from build123d import *

# Parameters (mm, degrees)
SKETCH1_R               = 5
BOSS_EXTRUDE1_DEPTH     = 5
SKETCH2_R               = 5.5
BOSS_EXTRUDE2_DEPTH     = 0.4
CUT_EXTRUDE1_DEPTH      = 6.4
SKETCH5_R               = 8
CUT_EXTRUDE2_DEPTH      = 6.5
CUT_EXTRUDE2_DEPTH_BACK = 6.5
CHAMFER4_SIZE           = 1
CHAMFER4_SIZE2          = 0.383864035


with BuildPart() as part:
    # Sketch1 → Boss-Extrude1 (new body)
    with BuildSketch(Plane(origin=(0, 0, 0), x_dir=(1, 0, 0), z_dir=(0, 1, 0))):
        Circle(SKETCH1_R)
    extrude(amount=BOSS_EXTRUDE1_DEPTH)

    # Sketch2 → Boss-Extrude2 (add)
    with BuildSketch(Plane(origin=(0, 5, 0), x_dir=(1, 0, 0), z_dir=(0, 1, 0))):
        Circle(SKETCH2_R)
    extrude(amount=BOSS_EXTRUDE2_DEPTH)

    # Sketch4 → Cut-Extrude1 (cut, through all)
    with BuildSketch(Plane(origin=(0, 5.4, 0), x_dir=(1, 0, 0), z_dir=(0, 1, 0))):
        with BuildLine():
            Line((2.295250379, 1.5), (2.295250379, -1.5))
            ThreePointArc((2.295250379, -1.5), (0, -3.795250379), (-2.295250379, -1.5))
            Line((-2.295250379, -1.5), (-2.295250379, 1.5))
            ThreePointArc((-2.295250379, 1.5), (0, 3.795250379), (2.295250379, 1.5))
        make_face()
    extrude(amount=-CUT_EXTRUDE1_DEPTH, mode=Mode.SUBTRACT)

    # Sketch5 → Cut-Extrude2 (cut, two sides)
    with BuildSketch(Plane(origin=(0, 0, 0), x_dir=(0, 0, -1), z_dir=(1, 0, 0))) as cut_extrude2_sk:
        with Locations((1, -3)):
            Circle(SKETCH5_R)
    extrude(amount=CUT_EXTRUDE2_DEPTH, mode=Mode.SUBTRACT)
    extrude(cut_extrude2_sk.sketch, amount=-CUT_EXTRUDE2_DEPTH_BACK, mode=Mode.SUBTRACT)

    # Chamfer4
    chamfer4_edges = [part.edges().sort_by_distance(p)[0] for p in [
        (0, 5.4, -3.795250379),
        (-2.295250379, 5.4, 0),
        (0, 5.4, 3.795250379),
        (2.295250379, 5.4, 0),
    ]]
    chamfer4_side = [part.faces().sort_by_distance(p)[0] for p in [
        (-5.344436508, 5.4, 0),
    ]]
    chamfer(chamfer4_edges, length=CHAMFER4_SIZE, length2=CHAMFER4_SIZE2, reference=chamfer4_side[0])


solid = part.part
Can you work these out from the model? Positions are in its coordinate system, mm. A direction names the side the tool comes from. Give positions to 0.01 mm unless a question says otherwise; leave off trailing zeros. Loops run counter-clockwise (first coordinate to the right, second up) from the corner with the lowest first, then second, coordinate; pieces in that order, holes last. Notation, with made-up numbers: (9.5, 54.5) - (46.5, 54.5) arc R27 cw to (46.5, 71.5) - close; hole circle Ø2 at (17.5, 46). An arc over 180 degrees is marked (long way). Answer as a JSON object with one key per item and string values.
Q1. Imagine slicing it at D-D on y = 3.2. Write out the boundary of the cut face in (x, z), plus the area to 3 significant figures.
Geometry says:
{"outline": "(-2.92, 4.06) - (2.92, 4.06) arc R5 ccw to start", "area": "3.76 mm²"}
Q2. Imagine slicing it at A-A on x = 0. Write out the boundary of the cut face in (y, z).
Geometry says:
{"outline": "(2.29, 5) arc R8 cw to (3.4, 3.8) - (5.02, 3.8) - (5.4, 4.8) - (5.4, 5.5) - (5, 5.5) - (5, 5) - close; (3.93, -5) - (5, -5) - (5, -5.5) - (5.4, -5.5) - (5.4, -4.8) - (5.02, -3.8) - (4.5, -3.8) arc R8 cw to start"}
Q3. Which directions (+Z, -Z, +X, -X, +Y, -Y) give clear straight access to the entire face, cutting with the end or side of a thin tool? Please do faces 1 (the cylindrical face through (0.1, 4.6, -5)), 2 (the cylindrical face through (0.05, 4.4, 3.795)), 3 (the flat face through (-2.788, 5.205, 0.021)), 4 (the flat face through (1.6, 5, 4.9)).
Geometry says:
{"face 1": "-Z, -Y", "face 2": "+Y, -Y", "face 3": "+Y", "face 4": "-Y"}
Q4. Imagine slicing it at B-B on z = 0. Write out the boundary of the cut face in (x, y), plus the area to 3 significant figures.
Geometry says:
{"outline": "(-5.5, 5) - (-5, 5) - (-5, 4.94) - (-2.3, 4.94) - (-2.3, 5.02) - (-3.3, 5.4) - (-5.5, 5.4) - close; (2.3, 4.94) - (5, 4.94) - (5, 5) - (5.5, 5) - (5.5, 5.4) - (3.3, 5.4) - (2.3, 5.02) - close", "area": "2.52 mm²"}
Q5. Imagine slicing it at C-C on y = 4.8. Write out the boundary of the cut face in (x, z).
Geometry says:
{"outline": "(-4.94, 0.78) - (-2.3, 0.78) - (-2.3, 1.5) arc R2.3 cw to (2.3, 1.5) - (2.3, 0.78) - (4.94, 0.78) arc R5 ccw to start; (-4.16, -2.78) arc R5 ccw to (4.16, -2.78) - (1.91, -2.78) arc R2.3 cw to (-1.91, -2.78) - close"}
Q6. If I drill on L1, parallel to Z at x = 1.5, y = 4.85; L2, parallel to Y at x = 2.5, z = 4.25; L3, parallel to Y at x = 3.25, z = 4, over which ranges is the centre line in solid material (lowest first)?
Geometry says:
{"L1": "-4.77 to -3.24, 3.24 to 4.77", "L2": "3.04 to 5.4", "L3": "5 to 5.4"}
Q7. Will these pins go through, and if not, where does the flat tip stop? P1, Ø0.5, axis at y = 5, z = 0.5, coming from the -X side; P2, Ø1, axis at x = 0, y = 4, coming from the +Z side; P3, Ø3.5, axis at x = -1, z = 2, coming from the -Y side.
Geometry says:
{"P1": "x = -5.49", "P2": "z = 5", "P3": "y = 3.44"}
